```python
from build123d import *

# Parameters (mm, degrees)
SKETCH_1_W      = 40.5
SKETCH_1_H      = 21
EXTRUDE_1_DEPTH = 32.45
SKETCH_2_W      = 7.3
SKETCH_2_H      = 21
SKETCH_2_R      = 2.25
EXTRUDE_2_DEPTH = 2.5
SKETCH_3_W      = 40
SKETCH_3_H      = 21
EXTRUDE_3_DEPTH = 9.6
SKETCH_4_R      = 3
EXTRUDE_4_DEPTH = 5.8


with BuildPart() as part:
    # 草图1 → 凸台-拉伸1 (new body)
    with BuildSketch(Plane(origin=(0, 0, 0), x_dir=(1, 0, 0), z_dir=(0, 1, 0))):
        Rectangle(SKETCH_1_W, SKETCH_1_H)
    extrude(amount=EXTRUDE_1_DEPTH)

    # 草图2 → 凸台-拉伸2 (add)
    # profile 1 of 2: a face of its own
    with BuildSketch(Plane(origin=(0, 32.45, 0), x_dir=(1, 0, 0), z_dir=(0, 1, 0))):
        with Locations((23.9, 0)):
            Rectangle(SKETCH_2_W, SKETCH_2_H)
        with Locations(Location((24, 5, 0), (0, 0, 270))):
            Circle(SKETCH_2_R, mode=Mode.SUBTRACT)
        with Locations(Location((24, -5, 0), (0, 0, 90))):
            Circle(SKETCH_2_R, mode=Mode.SUBTRACT)
    # profile 2 of 2: a face of its own
    with BuildSketch(Plane(origin=(0, 32.45, 0), x_dir=(1, 0, 0), z_dir=(0, 1, 0))):
        with Locations((-23.9, 0)):
            Rectangle(SKETCH_2_W, SKETCH_2_H)
        with Locations(Location((-24, -5, 0), (0, 0, 270))):
            Circle(SKETCH_2_R, mode=Mode.SUBTRACT)
        with Locations(Location((-24, 5, 0), (0, 0, 90))):
            Circle(SKETCH_2_R, mode=Mode.SUBTRACT)
    extrude(amount=-EXTRUDE_2_DEPTH)

    # 草图3 → 凸台-拉伸3 (add)
    with BuildSketch(Plane(origin=(0, 32.45, 0), x_dir=(1, 0, 0), z_dir=(0, 1, 0))):
        Rectangle(SKETCH_3_W, SKETCH_3_H)
    extrude(amount=EXTRUDE_3_DEPTH)

    # 草图4 → 凸台-拉伸4 (add)
    with BuildSketch(Plane(origin=(0, 42.05, 0), x_dir=(1, 0, 0), z_dir=(0, 1, 0))):
        with Locations(Location((-10, 0, 0), (0, 0, 90))):
            Circle(SKETCH_4_R)
    extrude(amount=EXTRUDE_4_DEPTH)


solid = part.part
```
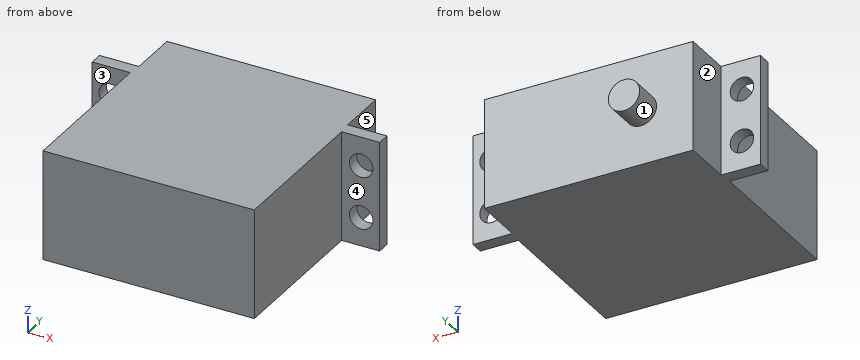
Build history of the part. All positions in model axes, mm. Face numbers are marked on the shaded views. A direction names the side the tool comes from. Coordinates: 2 decimals unless noted, no trailing zeros. Write each loop counter-clockwise with the first axis right and the second up, starting at its lowest first coordinate (ties: lowest second). Pieces come first, ordered by that corner, then holes.
1. Drop flat-ended pins along their axis: pin 1 (6 mm diameter, centred on x = -24, z = 1.5, fed in from +Y); pin 2 (10 mm diameter, centred on y = 35, z = -4, fed in from +X); pin 3 (5 mm diameter, centred on y = 22, z = -2, fed in from +X); pin 4 (3.5 mm diameter, centred on x = 25.5, z = 2.5, fed in from -Y). Give the stop position or say it passes through.
Answer block:
pin 1: stops at y = 32.45
pin 2: stops at x = 27.55
pin 3: stops at x = 20.25
pin 4: stops at y = 29.95
2. Band-saw the part on B-B, the plane z = 5. Give the cut face in (x, y).
Answer block:
outline: (-27.55, 29.95) - (-26.25, 29.95) - (-26.25, 32.45) - (-27.55, 32.45) - close; (-21.75, 29.95) - (-20.25, 29.95) - (-20.25, 0) - (20.25, 0) - (20.25, 29.95) - (21.75, 29.95) - (21.75, 32.45) - (20, 32.45) - (20, 42.05) - (-20, 42.05) - (-20, 32.45) - (-21.75, 32.45) - close; (26.25, 29.95) - (27.55, 29.95) - (27.55, 32.45) - (26.25, 32.45) - close
3. Drill centre lines: probe 1 along X at (y, z) = (30.8, -5); probe 2 along X at (y, z) = (5.5, 4.75); probe 3 along Y at (x, z) = (4, -8). Where is each one in solid material? Low to high.
Answer block:
probe 1: x = -27.55 to -26.25, -21.75 to 21.75, 26.25 to 27.55
probe 2: x = -20.25 to 20.25
probe 3: y = 0 to 42.05
4. Band-saw the part on A-A, the plane x = 24. Give the cut face in (y, z).
Answer block:
outline: (29.95, -10.5) - (32.45, -10.5) - (32.45, -7.25) - (29.95, -7.25) - close; (29.95, -2.75) - (32.45, -2.75) - (32.45, 2.75) - (29.95, 2.75) - close; (29.95, 7.25) - (32.45, 7.25) - (32.45, 10.5) - (29.95, 10.5) - close
5. Band-saw the part on D-D, the plane y = 37.5. Give the cut face in (x, z).
Answer block:
outline: (-20, -10.5) - (20, -10.5) - (20, 10.5) - (-20, 10.5) - close
6. Band-saw the part on C-C, the plane z = 0. Give the cut face in (x, y).
Answer block:
outline: (-27.55, 29.95) - (-20.25, 29.95) - (-20.25, 0) - (20.25, 0) - (20.25, 29.95) - (27.55, 29.95) - (27.55, 32.45) - (20, 32.45) - (20, 42.05) - (-7, 42.05) - (-7, 47.85) - (-13, 47.85) - (-13, 42.05) - (-20, 42.05) - (-20, 32.45) - (-27.55, 32.45) - close
7. 3-axis set-ups, long thin cutter, end or side, ignore diameter. For the marked faces 1, 2, 3, 4 and 5: which of +Z, -Z, +X, -X, +Y, -Y reach the whole face in a straight line?
Answer block:
face 1: +Y
face 2: +Z, -Z, -X, +Y
face 3: +Z, -Z, -X, -Y
face 4: +Z, -Z, +X, -Y
face 5: +Z, -Z, +X, +Y
